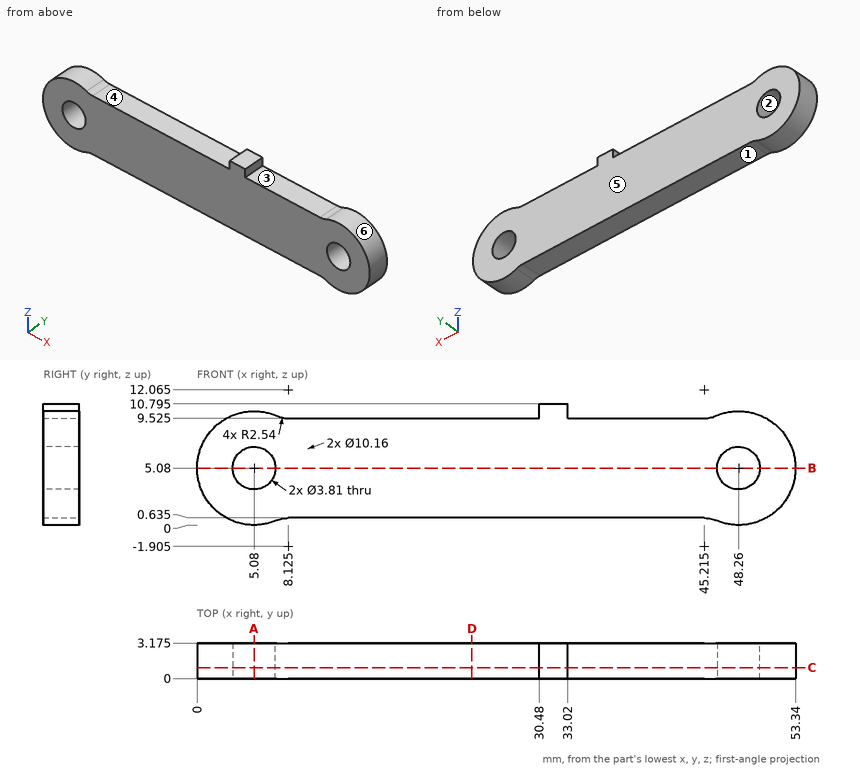
Here's the drawing with two shaded views (mm, measured from the low corner). I have some questions. A direction names the side the tool comes from. Round coordinates to 2 decimals unless told otherwise and drop trailing zeros. Loops run counter-clockwise (first coordinate to the right, second up) from the corner with the lowest first, then second, coordinate; pieces in that order, holes last. Notation, with made-up numbers: (79.5, 8) - (137.5, 8) arc R28 ccw to (137.5, 35) - close; hole circle Ø9 at (-21.5, 34.25). An arc over 180 degrees is marked (long way). Use CSV: the item, a comma, the result in double quotes.
Item 1: I need wall thicknesses on L1, parallel to X at y = 2.55, z = 5.08 (1 decimal); L2, parallel to Z at x = 5.08, y = 1.5 (1 decimal); L3, parallel to X at y = 2.9, z = 5.75 (1 decimal). Which ranges of each line are inside material? Lowest first, please. Write a range as [from, to].
Here are the results:
L1,"x = [0, 3.2], [7, 46.4], [50.2, 53.3]"
L2,"z = [0, 3.2], [7, 10.2]"
L3,"x = [0, 3.3], [6.9, 46.5], [50, 53.3]"
Item 2: If we section it at C-C on y = 1: List the corners of the cut face in (x, z) for me (1 decimal).
Here are the results:
outline,"(7.1, 0.4) arc R2.5 cw to (8.1, 0.6) - (45.2, 0.6) arc R2.5 cw to (46.2, 0.4) arc R5.1 ccw (long way) to (46.2, 9.7) arc R2.5 cw to (45.2, 9.5) - (33, 9.5) - (33, 10.8) - (30.5, 10.8) - (30.5, 9.5) - (8.1, 9.5) arc R2.5 cw to (7.1, 9.7) arc R5.1 ccw (long way) to start; hole circle Ø3.8 at (5.1, 5.1); hole circle Ø3.8 at (48.3, 5.1)"
Item 3: If we mould it in two halves opening along X, with no side actions, what happens to the marked faces 4, 5 and 6? For each: pulls with the +X half, pulls with the -X half, needs draft (parallel to the pull), parting line crosses it, or undercut.
Here are the results:
face 4,"undercut"
face 5,"needs draft"
face 6,"undercut"
Item 4: Will these pins go through, and if not, where does the flat tip stop? pin 1 (0.6 mm diameter, centred on y = 1.5, z = 10.5, fed in from -X); pin 2 (1.5 mm diameter, centred on x = 13.5, y = 3, fed in from +Z) (3 decimals); pin 3 (1.6 mm diameter, centred on x = 20, y = 1, fed in from -Z) (3 decimals).
Here are the results:
pin 1,"stops at x = 30.48"
pin 2,"stops at z = 9.525"
pin 3,"stops at z = 0.635"
Item 5: If we section it at B-B on z = 5.08: List the corners of the cut face in (x, y) for me (1 decimal).
Here are the results:
outline,"(0, 0) - (3.2, 0) - (3.2, 3.2) - (0, 3.2) - close; (7, 0) - (46.4, 0) - (46.4, 3.2) - (7, 3.2) - close; (50.2, 0) - (53.3, 0) - (53.3, 3.2) - (50.2, 3.2) - close"
Item 6: For the marked faces 1, 2 and 3, which set-ups out of +Z, -Z, +X, -X, +Y, -Y let a thin tool reach every point of the face, with its end or its side?
Here are the results:
face 1,"-Z, +Y, -Y"
face 2,"+Y, -Y"
face 3,"+Z, +Y, -Y"
Item 7: If we section it at D-D on x = 24.5: List the corners of the cut face in (y, z) for me (1 decimal), then the cut area to 3 significant figures.
Here are the results:
outline,"(0, 0.6) - (3.2, 0.6) - (3.2, 9.5) - (0, 9.5) - close"
area,"28.2 mm²"
Item 8: If we section it at A-A on x = 5.08: List the corners of the cut face in (y, z) for me (1 decimal).
Here are the results:
outline,"(0, 0) - (3.2, 0) - (3.2, 3.2) - (0, 3.2) - close; (0, 7) - (3.2, 7) - (3.2, 10.2) - (0, 10.2) - close"
